CAD build for the part. Positions are in the model's coordinates, mm. A direction names the side the tool comes from. Coordinates: 2 decimals unless noted, no trailing zeros. Loops run counter-clockwise (first coordinate to the right, second up) from the corner with the lowest first, then second, coordinate; pieces in that order, holes last. Notation, with made-up numbers: M -24,22 L 0,22 A30 ccw 0,53 Z; hole C 59,36 d10. An arc over 180 degrees is marked long. Answer as a JSON object with one key per item and string values. Group by question number.
```python
from build123d import *

# Parameters (mm, degrees)
BOSS_EXTRUDE1_DEPTH = 158.2
BOSS_EXTRUDE2_DEPTH = 24.5
CUT_EXTRUDE1_DEPTH  = 22


with BuildPart() as part:
    # Sketch2 → Boss-Extrude1 (new body)
    with BuildSketch(Plane(origin=(0, 0, 0), x_dir=(0, 0, -1), z_dir=(1, 0, 0))):
        with BuildLine():
            Line((0, 3), (0, 0))
            Line((0, 0), (19.270354352, 0))
            ThreePointArc((19.270354352, 0), (21.327514497, 1.580728698), (23.499214303, 3))
            Line((23.499214303, 3), (0, 3))
        make_face()
        with BuildLine():
            ThreePointArc((23.499214303, 3), (21.327514497, 1.580728698), (19.270354352, 0))
            Line((19.270354352, 0), (24.351351406, 0))
            ThreePointArc((24.351351406, 0), (27.318789972, 1.667701058), (30.451184901, 3))
            Line((30.451184901, 3), (23.499214303, 3))
        make_face()
        with BuildLine():
            ThreePointArc((51.548815099, 3), (54.681210028, 1.667701058), (57.648648594, 0))
            Line((57.648648594, 0), (62.729645648, 0))
            ThreePointArc((62.729645648, 0), (60.672485503, 1.580728698), (58.500785697, 3))
            Line((58.500785697, 3), (51.548815099, 3))
        make_face()
        with BuildLine():
            ThreePointArc((30.451184901, 3), (27.318789972, 1.667701058), (24.351351406, 0))
            Line((24.351351406, 0), (57.648648594, 0))
            ThreePointArc((57.648648594, 0), (54.681210028, 1.667701058), (51.548815099, 3))
            Line((51.548815099, 3), (30.451184901, 3))
        make_face()
        with BuildLine():
            Line((126.499214303, 3), (58.500785697, 3))
            ThreePointArc((58.500785697, 3), (60.672485503, 1.580728698), (62.729645648, 0))
            Line((62.729645648, 0), (122.270354352, 0))
            ThreePointArc((122.270354352, 0), (124.327514497, 1.580728698), (126.499214303, 3))
        make_face()
        with BuildLine():
            Line((133.451184901, 3), (126.499214303, 3))
            ThreePointArc((126.499214303, 3), (124.327514497, 1.580728698), (122.270354352, 0))
            Line((122.270354352, 0), (127.351351406, 0))
            ThreePointArc((127.351351406, 0), (130.318789972, 1.667701058), (133.451184901, 3))
        make_face()
        with BuildLine():
            ThreePointArc((165.729645648, 0), (163.672485503, 1.580728698), (161.500785697, 3))
            Line((161.500785697, 3), (154.548815099, 3))
            ThreePointArc((154.548815099, 3), (157.681210028, 1.667701058), (160.648648594, 0))
            Line((160.648648594, 0), (165.729645648, 0))
        make_face()
        with BuildLine():
            Line((154.548815099, 3), (133.451184901, 3))
            ThreePointArc((133.451184901, 3), (130.318789972, 1.667701058), (127.351351406, 0))
            Line((127.351351406, 0), (160.648648594, 0))
            ThreePointArc((160.648648594, 0), (157.681210028, 1.667701058), (154.548815099, 3))
        make_face()
        with BuildLine():
            Line((175, 3), (161.500785697, 3))
            ThreePointArc((161.500785697, 3), (163.672485503, 1.580728698), (165.729645648, 0))
            Line((165.729645648, 0), (175, 0))
            Line((175, 0), (175, 3))
        make_face()
    extrude(amount=-BOSS_EXTRUDE1_DEPTH)

    # Sketch2_5 → Boss-Extrude2 (add)
    with BuildSketch(Plane(origin=(0, 0, 0), x_dir=(0, 0, -1), z_dir=(1, 0, 0))):
        with BuildLine():
            ThreePointArc((58.500785697, 3), (41, 7.85), (23.499214303, 3))
            Line((23.499214303, 3), (30.451184901, 3))
            ThreePointArc((30.451184901, 3), (41, 4.85), (51.548815099, 3))
            Line((51.548815099, 3), (58.500785697, 3))
        make_face()
        with BuildLine():
            ThreePointArc((51.548815099, 3), (41, 4.85), (30.451184901, 3))
            Line((30.451184901, 3), (51.548815099, 3))
        make_face()
        with BuildLine():
            ThreePointArc((161.500785697, 3), (144, 7.85), (126.499214303, 3))
            Line((126.499214303, 3), (133.451184901, 3))
            ThreePointArc((133.451184901, 3), (144, 4.85), (154.548815099, 3))
            Line((154.548815099, 3), (161.500785697, 3))
        make_face()
        with BuildLine():
            ThreePointArc((154.548815099, 3), (144, 4.85), (133.451184901, 3))
            Line((133.451184901, 3), (154.548815099, 3))
        make_face()
    boss_extrude2 = extrude(amount=-BOSS_EXTRUDE2_DEPTH)

    # Sketch2_7 → Cut-Extrude1 (cut)
    with BuildSketch(Plane(origin=(0, 0, 0), x_dir=(0, 0, -1), z_dir=(1, 0, 0))):
        with BuildLine():
            ThreePointArc((30.451184901, 3), (27.318789972, 1.667701058), (24.351351406, 0))
            Line((24.351351406, 0), (57.648648594, 0))
            ThreePointArc((57.648648594, 0), (54.681210028, 1.667701058), (51.548815099, 3))
            Line((51.548815099, 3), (30.451184901, 3))
        make_face()
        with BuildLine():
            ThreePointArc((51.548815099, 3), (41, 4.85), (30.451184901, 3))
            Line((30.451184901, 3), (51.548815099, 3))
        make_face()
        with BuildLine():
            Line((154.548815099, 3), (133.451184901, 3))
            ThreePointArc((133.451184901, 3), (130.318789972, 1.667701058), (127.351351406, 0))
            Line((127.351351406, 0), (160.648648594, 0))
            ThreePointArc((160.648648594, 0), (157.681210028, 1.667701058), (154.548815099, 3))
        make_face()
        with BuildLine():
            ThreePointArc((154.548815099, 3), (144, 4.85), (133.451184901, 3))
            Line((133.451184901, 3), (154.548815099, 3))
        make_face()
    cut_extrude1 = extrude(amount=-CUT_EXTRUDE1_DEPTH, mode=Mode.SUBTRACT)

    # Mirror1: Boss-Extrude2, Cut-Extrude1 across plane
    add(boss_extrude2.mirror(Plane(origin=(-79.1, 0, 0), x_dir=(0, 0, 1), z_dir=(1, 0, 0))))
    add(cut_extrude1.mirror(Plane(origin=(-79.1, 0, 0), x_dir=(0, 0, 1), z_dir=(1, 0, 0))), mode=Mode.SUBTRACT)


solid = part.part
```
Item 1: Slice it at C-C, the plane x = -96. Write the cut outline in (y, z), then the cut area to 3 significant figures.
Item 2: Pin check, flat tips, straight feed: pin 1 (2 mm diameter, centred on x = -46, z = -73, fed in from +Y); pin 2 (2.5 mm diameter, centred on y = 3, z = -147.5, fed in from -X); pin 3 (3 mm diameter, centred on y = 5, z = -74.5, fed in from -X). Stop position of each tip, or through.
Item 3: Drill centre lines: L1, parallel to X at y = 3.5, z = -159.5; L2, parallel to Y at x = -50, z = -89; L3, parallel to Y at x = -143, z = -41. Where is each one in solid material? Low to high. Write a range as from..to.
Item 4: Pull direction Z, two halves, no side cores. Call faces 5 (the cylindrical face through (-146.12, 7.85, -41.26)), 6 (the flat face through (-136.2, 2, -41)), 7 (the flat face through (-133.7, 5, -144)): released by +Z, released by -Z, zero draft, split by the parting line, or undercut.
Item 5: Tool access for faces 1 (the flat face through (-78, 0, -86)), 2 (the flat face through (-136.2, 2, -144)), 3 (the flat face through (-133.7, 5, -41)), 4 (the flat face through (-22, 2, -41)): list every direction of +Z, -Z, +X, -X, +Y, -Y with a clear straight run to the whole face (end or side of a thin tool).
Item 6: Slice it at B-B, the plane z = -144. Write the cut outline in (x, y), then the cut area to 3 significant figures.
Item 7: Slice it at A-A, the plane x = -9.5. Write the cut outline in (y, z), then the cut area to 3 significant figures.
Computed:
{
 "1": {"outline": "M 0,-175 L 3,-175 L 3,0 L 0,0 Z", "area": "525 mm2"},
 "2": {"pin 1": "y = 3", "pin 2": "x = -136.2", "pin 3": "through"},
 "3": {"L1": "-158.2..-133.7, -24.5..0", "L2": "0..3", "L3": "4.85..7.85"},
 "4": {"face 5": "undercut", "face 6": "undercut", "face 7": "zero draft"},
 "5": {"face 1": "+Z, -Z, +X, -X, -Y", "face 2": "-X, -Y", "face 3": "+Z, -Z, +Y", "face 4": "+X, -Y"},
 "6": {"outline": "M -158.2,4.85 L -136.2,4.85 L -136.2,0 L -22,0 L -22,4.85 L 0,4.85 L 0,7.85 L -24.5,7.85 L -24.5,3 L -133.7,3 L -133.7,7.85 L -158.2,7.85 Z", "area": "499 mm2"},
 "7": {"outline": "M 0,-175 L 3,-175 L 3,-161.5 A34 ccw 3,-126.5 L 3,-58.5 A34 ccw 3,-23.5 L 3,0 L 0,0 L 0,-24.35 A31 cw 0,-57.65 L 0,-127.35 A31 cw 0,-160.65 Z", "area": "536 mm2"}
}
